Could you check a few things on this model? Use its own coordinates, in mm. A direction names the side the tool comes from. Round coordinates to 2 decimals unless told otherwise and drop trailing zeros. Write each loop counter-clockwise with the first axis right and the second up, starting at its lowest first coordinate (ties: lowest second). Pieces come first, ordered by that corner, then holes. Notation, with made-up numbers: (53.5, 74.5) -> (105.5, 74.5) arc R32 ccw to (105.5, 106.5) -> close; hole circle Ø5 at (-12.5, -1.5). An arc over 180 degrees is marked (long way). One line per question, with ' | ' between items. Start each with the question number.
1. If I drill on line 1 along Z through (x, y) = (3, 1.1) (3 decimals); line 2 along X through (y, z) = (0.4, -44.5); line 3 along X through (y, z) = (0.75, -19), over which ranges is the centre line in solid material (lowest first)? Write a range as [from, to].
2. Imagine slicing it at D-D, the plane x = 30. List the corners of the cut face in (y, z) for me (1 decimal).
3. For faces 1 (the flat face through (29.5, 1, -46)), 2 (the flat face through (19.5, 1, -2)), 3 (the flat face through (19.5, 1, -46)), which set-ups out of +Z, -Z, +X, -X, +Y, -Y let a thin tool reach every point of the face, with its end or its side?
4. Imagine slicing it at C-C, the plane z = -26. List the corners of the cut face in (x, y) for me.
5. Imagine slicing it at A-A, the plane x = 2.5. State how many separate pieces and enclosed holes the cut face has, and give its area (3 significant figures).
6. For pin 1 Ø0.5 at (y, z) = (0.5, -2.5) entering from +X; pin 2 Ø0.8 at (y, z) = (1, -22) entering from +X; pin 3 Ø1 at (x, z) = (9.5, -12.5) entering from -Y; pin 4 Ø0.8 at (x, y) = (36, 0.5) entering from +Z (3 decimals), each with a flat end and sliding along its axis, tell me the tip position at first contact or that it passes through.
7. Thinking about a two-plate mould opening in Z: for faces 4 (the flat face through (37.175, 1, -34)), 5 (the flat face through (2, 1, -8.675)), 6 (the flat face through (32, 1, -44.175)), which applies, released by +Z, released by -Z, zero draft, split by the parting line, or undercut?
from build123d import *

# Parameters (mm, degrees)
SKETCH1_W           = 37.175
SKETCH1_H           = 47.35
BOSS_EXTRUDE1_DEPTH = 1.5875
SKETCH2_W           = 3.175
SKETCH2_H           = 10
SKETCH2_H_2         = 5.5
SKETCH2_W_2         = 10
SKETCH2_H_3         = 3.175
CUT_EXTRUDE1_DEPTH  = 2.5875


with BuildPart() as part:
    # Sketch1 → Boss-Extrude1 (new body)
    with BuildSketch(Plane(origin=(0, 0, 0), x_dir=(1, 0, 0), z_dir=(0, 1, 0))):
        with Locations((18.5875, 23.675)):
            Rectangle(SKETCH1_W, SKETCH1_H)
    extrude(amount=BOSS_EXTRUDE1_DEPTH)

    # Sketch2 → Cut-Extrude1 (cut, through all)
    with BuildSketch(Plane(origin=(0, 1.5875, 0), x_dir=(1, 0, 0), z_dir=(0, 1, 0))):
        Polygon((37.175, 47.35), (29.5, 47.35), (29.5, 44.175), (34, 44.175), (34, 38.675), (37.175, 38.675), align=None)
        with Locations((35.5875, 23.675)):
            Rectangle(SKETCH2_W, SKETCH2_H)
        Polygon((29.5, 3.175), (29.5, 0), (37.175, 0), (37.175, 3.175), (34, 3.175), align=None)
        with Locations((35.5875, 5.925)):
            Rectangle(SKETCH2_W, SKETCH2_H_2)
        with Locations((14.5, 1.5875)):
            Rectangle(SKETCH2_W_2, SKETCH2_H_3)
        with Locations((1.5875, 13.675)):
            Rectangle(SKETCH2_W, SKETCH2_H)
        with Locations((1.5875, 33.675)):
            Rectangle(SKETCH2_W, SKETCH2_H)
        with Locations((14.5, 45.7625)):
            Rectangle(SKETCH2_W_2, SKETCH2_H_3)
    extrude(amount=-CUT_EXTRUDE1_DEPTH, mode=Mode.SUBTRACT)


solid = part.part
Geometry results:
1) line 1: z = [-47.35, -38.675], [-28.675, -18.675], [-8.675, 0] | line 2: x = [0, 9.5], [19.5, 29.5] | line 3: x = [0, 34]
2) outline: (0, -44.2) -> (1.6, -44.2) -> (1.6, -3.2) -> (0, -3.2) -> close
3) face 1: -Z, +X, +Y, -Y | face 2: +Z, +Y, -Y | face 3: -Z, +Y, -Y
4) outline: (0, 0) -> (34, 0) -> (34, 1.59) -> (0, 1.59) -> close
5) separate pieces: 3 | enclosed holes: 0 | area: 43.4 mm2
6) pin 1: stops at x = 29.5 | pin 2: stops at x = 34 | pin 3: stops at y = 0 | pin 4: stops at z = -8.675
7) face 4: zero draft | face 5: undercut | face 6: released by -Z
